Autodesk Fusion 360 part; units mm, degrees
sketch "Sketch1" plane through (0, 0, 0) normal (0, 1, 0) x (1, 0, 0)
  circle A0 centre (0, 0) radius 5
  circle A1 centre (0, 0) radius 4
  dimension "d1" = 10
  dimension "d2" = 8
extrude "Extrude1" add sketch "Sketch1" along normal blind 160
sketch "Sketch2" plane through (0, 0, 0) normal (0, 0, 1) x (1, 0, 0)
  line L0 (-5, 0) -> (5, 0)
  line L1 (5, 0) -> (5, 15)
  line L2 (5, 15) -> (-5, 15)
  line L3 (-5, 15) -> (-5, 0)
  line L4 (-5, 15) -> (5, 15)
  line L5 (5, 15) -> (5, 25)
  line L6 (5, 25) -> (-5, 25)
  line L7 (-5, 25) -> (-5, 15)
  line L8 (-5, 25) -> (-2.5, 25)
  line L9 (-2.5, 25) -> (-2.5, 15)
  line L10 (-2.5, 15) -> (-5, 15)
  line L11 (-5, 15) -> (-5, 25)
  line L12 (5, 15) -> (2.5, 15)
  line L13 (2.5, 15) -> (2.5, 25)
  line L14 (2.5, 25) -> (5, 25)
  line L15 (5, 25) -> (5, 15)
  dimension "d5" = 10
  dimension "d6" = 15
  dimension "d7" = 10
  dimension "d8" = 10
  dimension "d9" = 2.5
  dimension "d10" = 10
  dimension "d11" = 2.5
  dimension "d12" = 10
extrude "Extrude2" cut sketch "Sketch2" along normal mid plane 20 contours L2 L4 L6 L7 L8 L9 L10 L11 | L2 L4 L5 L6 L12 L13 L14 L15
equation "d2 = d1 - 2 mm"
equation "d5 = d1"
equation "d7 = d1"
equation "d9 = d1 / 4"
equation "d10 = d1"
equation "d11 = d1 / 4"
equation "d12 = d1"
equation "d13 = d1"
Read the model definition and answer for the solid it produces. Units are mm, in the model's axes. A direction names the side the tool comes from. Round coordinates to 2 decimals unless told otherwise and drop trailing zeros. Write each loop counter-clockwise with the first axis right and the second up, starting at its lowest first coordinate (ties: lowest second). Pieces come first, ordered by that corner, then holes.
Q1. A tool of negligible diameter and unlimited length cuts with its end or side. For faces 4 (the face through (-4.3, 15, -0.1)), 5 (the face through (4.3, 25, -0.1)), from which of +Z, -Z, +X, -X, +Y, -Y can it reach the whole face along a straight path? Write none if from no direction.
Values:
face 4: +Z, -Z, -X
face 5: +Z, -Z, +X
Q2. Find section D-D on y = 119. Determine the outline of the cut face in (x, z), and give its area (3 significant figures).
Values:
outline: circle Ø10 at (0, 0); hole circle Ø8 at (0, 0)
area: 28.3 mm2
Q3. Find section A-A on z = 0. Determine the outline of the cut face in (x, y).
Values:
outline: (-5, 0) - (-4, 0) - (-4, 15) - (-5, 15) - close; (-5, 25) - (-4, 25) - (-4, 160) - (-5, 160) - close; (4, 0) - (5, 0) - (5, 15) - (4, 15) - close; (4, 25) - (5, 25) - (5, 160) - (4, 160) - close
Q4. Find section C-C on x = 0. Determine the outline of the cut face in (y, z), and give its area (3 significant figures).
Values:
outline: (0, -5) - (160, -5) - (160, -4) - (0, -4) - close; (0, 4) - (160, 4) - (160, 5) - (0, 5) - close
area: 320 mm2
Q5. Straight lines are drawn through the part: line 1 (X direction, y = 96, z = 0); line 2 (Y direction, x = 2.75, z = -3.5); line 3 (Z direction, x = -2.5, y = 12). For each, find the intervals that lie inside material, in ascending order.
Values:
line 1: x = -5 to -4, 4 to 5
line 2: y = 0 to 15, 25 to 160
line 3: z = -4.33 to -3.12, 3.12 to 4.33
Q6. The mould has two halves that part along Z. Classify faces 1 (the face through (-1.08, 78.88, -4.88)), 2 (the face through (-4.3, 25, -0.1)), 3 (the face through (-0.867, 78.88, -3.905)): released by +Z, released by -Z, zero draft, split by the parting line, or undercut.
Values:
face 1: split by the parting line
face 2: zero draft
face 3: undercut
Q7. Flat-ended cylindrical pins translate along their axes: P1, Ø1, axis at y = 22, z = -3.5, coming from the -X side; P2, Ø2, axis at y = 82.5, z = -2, coming from the +X side; P3, Ø2, axis at x = 3, y = 126.5, coming from the -Z side. Find the tip coordinate at first contact, or state that the pin passes through.
Values:
P1: stops at x = -2.5
P2: stops at x = 4.9
P3: stops at z = -4.58
Q8. Find section B-B on y = 21.5. Determine the outline of the cut face in (x, z), and give its area (3 significant figures).
Values:
outline: (-2.5, -4.33) arc R5 ccw to (2.5, -4.33) - (2.5, -3.12) arc R4 cw to (-2.5, -3.12) - close; (-2.5, 3.12) arc R4 cw to (2.5, 3.12) - (2.5, 4.33) arc R5 ccw to (-2.5, 4.33) - close
area: 10.6 mm2
